Build history of the part. All positions in model axes, mm. Face numbers are marked on the shaded views. A direction names the side the tool comes from. Coordinates: 2 decimals unless noted, no trailing zeros. Write each loop counter-clockwise with the first axis right and the second up, starting at its lowest first coordinate (ties: lowest second). Pieces come first, ordered by that corner, then holes.
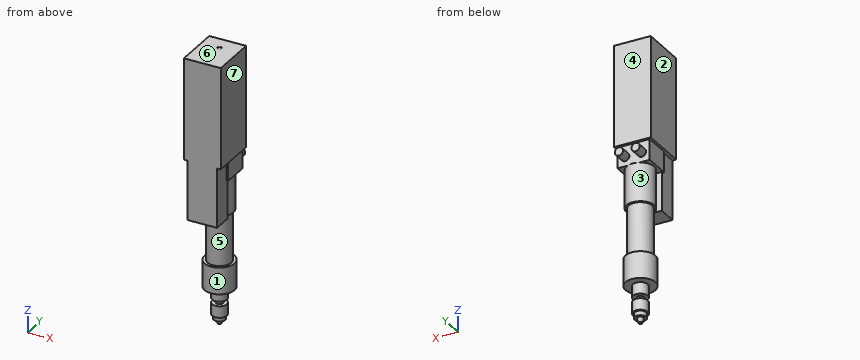
```python
from build123d import *

# Parameters (mm, degrees)
F0_R           = 32.5
F1_DEPTH       = 58
F2_R           = 16
F3_DEPTH       = 25
F4_R           = 26
F5_DEPTH       = 110
F6_R           = 30
F7_DEPTH       = 84
F8_W           = 70
F8_H           = 57
F9_DEPTH       = 85
F10_W          = 64
F10_H          = 42
F11_DEPTH      = 169
F12_W          = 80
F12_H          = 100
F13_DEPTH      = 180
F13_DEPTH_BACK = 40
F14_R          = 9
F15_DEPTH      = 25
F16_R          = 7.5
F17_DEPTH      = 10
F18_R          = 16
F19_DEPTH      = 25
F20_R          = 12.5
F21_DEPTH      = 10
F24_R          = 5
F25_DEPTH      = 1


with BuildPart() as f1:
    # F0 (on Top) → F1 (new body)
    with BuildSketch(Plane.XY):
        Circle(F0_R)
    extrude(amount=-F1_DEPTH)

    # F4 (on Top) → F5 (join)
    with BuildSketch(Plane.XY):
        Circle(F4_R)
    extrude(amount=F5_DEPTH)

    # F6 (on face) → F7 (join)
    with BuildSketch(Plane.XY.offset(110)):
        Circle(F6_R)
    extrude(amount=F7_DEPTH)

    # F8 (on face) → F9 (join)
    with BuildSketch(Plane.XY.offset(194)):
        with Locations((0, -1.5)):
            Rectangle(F8_W, F8_H)
    extrude(amount=F9_DEPTH)

    # F10 (on face) → F11 (join, through all)
    with BuildSketch(Plane(origin=(0, 0, 110), x_dir=(1, 0, 0), z_dir=(0, 0, -1))):
        with Locations((0, 47)):
            Rectangle(F10_W, F10_H)
    extrude(amount=-F11_DEPTH)

    # F12 (on face) → F13 (join, two sides)
    with BuildSketch(Plane.XY.offset(279)) as f13_sk:
        with Locations((0, -18)):
            Rectangle(F12_W, F12_H)
    extrude(amount=F13_DEPTH)
    extrude(f13_sk.sketch, amount=-F13_DEPTH_BACK)

    # F14 (on face) → F15 (join)
    with BuildSketch(Plane(origin=(0, 27, 0), x_dir=(-1, 0, 0), z_dir=(0, 1, 0))):
        with Locations((18, 214)):
            Circle(F14_R)
        with Locations((-18, 214)):
            Circle(F14_R)
    extrude(amount=F15_DEPTH)



with BuildPart() as f3:
    # F2 (on face) → F3 (new body)
    with BuildSketch(Plane(origin=(0, 0, -93), x_dir=(1, 0, 0), z_dir=(0, 0, -1))):
        Circle(F2_R)
    extrude(amount=F3_DEPTH)

    # F16 (on face) → F17 (join)
    with BuildSketch(Plane(origin=(0, 0, -83), x_dir=(1, 0, 0), z_dir=(0, 0, -1))):
        Circle(F16_R)
    extrude(amount=F17_DEPTH)


with BuildPart() as f1_1:
    add(f1.part)

    add(f3.part)  # F19 merges F3
    # F18 (on face) → F19 (join)
    with BuildSketch(Plane(origin=(0, 0, -58), x_dir=(1, 0, 0), z_dir=(0, 0, -1))):
        Circle(F18_R)
    extrude(amount=F19_DEPTH)

    # F20 (on face) → F21 (join)
    with BuildSketch(Plane(origin=(0, 0, -118), x_dir=(1, 0, 0), z_dir=(0, 0, -1))):
        Circle(F20_R)
    extrude(amount=F21_DEPTH)

    # F22 (on Front) → F23 (revolve)
    with BuildSketch(Plane.XZ):
        Polygon((0, -138), (0, -128), (-7, -128), (-4, -138), align=None)
    revolve(axis=Axis((0, 0, -93), (0, 0, 1)))

    # F24 (on face) → F25 (cut)
    with BuildSketch(Plane.XY.offset(459)):
        Circle(F24_R)
    extrude(amount=-F25_DEPTH, mode=Mode.SUBTRACT)


solid = f1_1.part
```
1. Probe line 1 along Y through (x, z) = (0, 458.4); line 2 along Z through (x, y) = (9, 12); line 3 along Z through (x, y) = (22, 23). List the from-to ranges inside material, lowest first.
Computed values:
line 1: y = -68 to -5, 5 to 32
line 2: z = -118 to -93, -83 to 459
line 3: z = -58 to 0, 194 to 459
2. Saw through at C-C on y = -41. List the corners of the cut face in (x, z), plus the area to 3 significant figures.
Computed values:
outline: (-40, 239) - (-32, 239) - (-32, 110) - (32, 110) - (32, 239) - (40, 239) - (40, 459) - (-40, 459) - close
area: 25,900 mm2
3. Mould opens along Z. For the marked faces 5, 6 and 7 say: +Z half, -Z half, draft (parallel to the pull), parting line (faces both ways), or undercut.
Computed values:
face 5: undercut
face 6: +Z half
face 7: draft
4. 3-axis set-ups, long thin cutter, end or side, ignore diameter. For the marked faces 1, 2, 3 and 4: which of +Z, -Z, +X, -X, +Y, -Y reach the whole face in a straight line?
Computed values:
face 1: -Z
face 2: +Z, -Z, -X, +Y, -Y
face 3: none
face 4: +Z, +X, -X, +Y
5. Saw through at A-A on z = 214. List the corners of the cut face in (x, y), plus the area to 3 significant figures.
Computed values:
outline: (-35, -30) - (-32, -30) - (-32, -68) - (32, -68) - (32, -30) - (35, -30) - (35, 27) - (27, 27) - (27, 52) - (9, 52) - (9, 27) - (-9, 27) - (-9, 52) - (-27, 52) - (-27, 27) - (-35, 27) - close
area: 7,320 mm2
6. Saw through at B-B on y = 37.5. List the corners of the cut face in (x, z).
Computed values:
outline: circle Ø18 at (-18, 214); circle Ø18 at (18, 214)
7. Flat gauge pins, fed straight in: pin 1 (5 mm diameter, centred on x = -17.5, y = 18.5, fed in from -Z); pin 2 (2 mm diameter, centred on x = -15, z = 153.5, fed in from +Y); pin 3 (10 mm diameter, centred on y = -9, z = 140, fed in from +X). Where does each tip first touch, or does it go through?
Computed values:
pin 1: stops at z = -58
pin 2: stops at y = 26.53
pin 3: stops at x = 29.73
